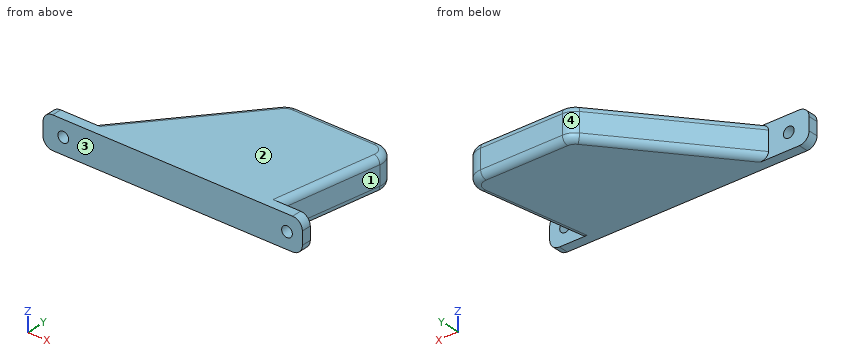
from build123d import *

# Parameters (mm, degrees)
BOSS_EXTRUDE1_DEPTH = 10
BOSS_EXTRUDE2_DEPTH = 3
FILLET2_R           = 3
SKETCH3_R           = 1.65
CUT_EXTRUDE2_DEPTH  = 80.806014811
FILLET4_R           = 5
FILLET3_R           = 2


with BuildPart() as part:
    # Sketch1 → Boss-Extrude1 (new body)
    with BuildSketch(Plane.XY):
        Polygon((0, 0), (60, 0), (67.053079228, 40), (33.563985247, 40), align=None)
    extrude(amount=BOSS_EXTRUDE1_DEPTH)

    # Sketch2 → Boss-Extrude2 (add)
    with BuildSketch(Plane.XZ):
        Polygon((0, 10), (-10, 10), (-10, 0), (0, 0), (70, 0), (70, 10), (60, 10), align=None)
    extrude(amount=-BOSS_EXTRUDE2_DEPTH)

    # Fillet2
    fillet2_edges = [part.edges().sort_by_distance(p)[0] for p in [
        (70, 1.5, 0),
        (-10, 1.5, 10),
        (70, 1.5, 10),
        (-10, 1.5, 0),
    ]]
    fillet(fillet2_edges, radius=FILLET2_R)

    # Sketch3 → Cut-Extrude2 (cut, through all)
    with BuildSketch(Plane(origin=(0, 3, 0), x_dir=(1, 0, 0), z_dir=(0, 1, 0))):
        with Locations(Location((65.264490471, -5, 0), (0, 0, 270))):
            Circle(SKETCH3_R)
        with Locations(Location((-3.741350553, -5, 0), (0, 0, 270))):
            Circle(SKETCH3_R)
    extrude(amount=-CUT_EXTRUDE2_DEPTH, mode=Mode.SUBTRACT)

    # Fillet4
    fillet4_edges = [part.edges().sort_by_distance(p)[0] for p in [
        (67.053079228, 40, 5),
        (33.563985247, 40, 5),
    ]]
    fillet(fillet4_edges, radius=FILLET4_R)

    # Fillet3
    fillet3_edges = [part.edges().sort_by_distance(p)[0] for p in [
        (63.273665486, 18.565879556, 0),
        (17.291300108, 20.606969024, 0),
        (17.291300108, 20.606969024, 10),
        (63.273665486, 18.565879556, 10),
        (48.494917402, 40, 0),
        (48.494917402, 40, 10),
        (33.782432229, 39.531538935, 0),
        (64.924533481, 38.213938048, 0),
        (33.782432229, 39.531538935, 10),
        (64.924533481, 38.213938048, 10),
    ]]
    fillet(fillet3_edges, radius=FILLET3_R)


solid = part.part
Model file for the job. Use its own axes, mm. Face numbers are marked on the shaded views. Give positions to 0.01 mm unless a question says otherwise; leave off trailing zeros. Write each loop counter-clockwise with the first axis right and the second up, starting at its lowest first coordinate (ties: lowest second). Pieces come first, ordered by that corner, then holes. Notation, with made-up numbers: (-5.5, -1) -> (47.5, -1) arc R22 ccw to (47.5, 35) -> close; hole circle Ø7 at (0, 73). An arc over 180 degrees is marked (long way). Write item = value, one per line.
(1) Flat gauge pins, fed straight in: P1, Ø1.5, axis at x = 24.5, z = 8.5, coming from the +Y side; P2, Ø3, axis at x = 18.5, y = 23, coming from the +Z side; P3, Ø2, axis at x = 65.26, z = 5, coming from the +Y side. Where does each tip first touch, or does it go through?
Determined:
P1 = 30.03
P2 = 9.66
P3 = 38.87
(2) Mould opens along Y. For the marked faces 1, 2, 3 and 4 say: released by +Y, released by -Y, zero draft, split by the parting line, or undercut.
Determined:
face_1 = undercut
face_2 = zero draft
face_3 = released by -Y
face_4 = released by +Y
(3) Slice it at B-B, the plane x = 0. Give the cut face in (y, z).
Determined:
outline = (0, 0) -> (3, 0) -> (3, 10) -> (0, 10) -> close
(4) Slice it at A-A, the plane z = 5. Give the cut face in (x, y).
Determined:
outline = (-10, 0) -> (-5.39, 0) -> (-5.39, 3) -> (-10, 3) -> close; (-2.09, 0) -> (63.61, 0) -> (63.61, 3) -> (60.53, 3) -> (66.02, 34.13) arc R5 ccw to (61.09, 40) -> (35.9, 40) arc R5 ccw to (32.07, 38.21) -> (2.52, 3) -> (-2.09, 3) -> close; (66.91, 0) -> (70, 0) -> (70, 3) -> (66.91, 3) -> close
(5) Slice it at C-C, the plane z = 1. Give the cut face in (x, y).
Determined:
outline = (-9.24, 0) -> (69.24, 0) -> (69.24, 3) -> (60.26, 3) -> (65.75, 34.18) arc R4.73 ccw to (61.09, 39.73) -> (35.9, 39.73) arc R4.73 ccw to (32.27, 38.04) -> (2.87, 3) -> (-9.24, 3) -> close
(6) Probe line 1 along X through (y, z) = (1.2, 5); line 2 along Y through (x, z) = (0, 5); line 3 along Y through (x, z) = (31, 5.25). List the from-to ranges inside material, lowest first.
Determined:
line_1 = -10 to -5.39, -2.09 to 63.61, 66.91 to 70
line_2 = 0 to 3
line_3 = 0 to 36.94
